Verification items for the finished model (mm, model axes). A direction names the side the tool comes from. Give positions to 0.01 mm unless a question says otherwise; leave off trailing zeros. Write each loop counter-clockwise with the first axis right and the second up, starting at its lowest first coordinate (ties: lowest second). Pieces come first, ordered by that corner, then holes. Notation, with made-up numbers: (8.25, -11.75) -> (44.25, -11.75) arc R22 ccw to (44.25, -0.75) -> close; hole circle Ø11 at (16, 11.25). An arc over 180 degrees is marked (long way). Answer as CSV lines item,"result".
```python
from build123d import *

# Parameters (mm, degrees)
SKETCH2_R          = 1.27
CUT_EXTRUDE1_DEPTH = 27.94
SKETCH3_R          = 2.54
CUT_EXTRUDE5_DEPTH = 2.54
CIRPATTERN1_COUNT  = 5


with BuildPart() as part:
    # Sketch1 → Revolve1 (revolve)
    with BuildSketch(Plane.YZ, mode=Mode.PRIVATE) as revolve1_sk:
        Polygon((0, 33.880456026), (-45.72, 33.880456026), (-45.72, 14.830456026), (-38.1, 14.830456026), (-38.1, 2.130456026), (0, 2.130456026), align=None)
    revolve(revolve1_sk.sketch.rotate(Axis((0, 0, 48.959120521), (0, 0, -1)), 270), axis=Axis((0, 0, 48.959120521), (0, 0, -1)))

    # Sketch2 → Cut-Extrude1 (cut)
    with BuildSketch(Plane.XY.offset(33.880456026)):
        with Locations((0, 41.91)):
            Circle(SKETCH2_R)
    cut_extrude1 = extrude(amount=-CUT_EXTRUDE1_DEPTH, mode=Mode.SUBTRACT)

    # Sketch3 → Cut-Extrude5 (cut)
    with BuildSketch(Plane.XY.offset(33.880456026)):
        with Locations((0, 41.91)):
            Circle(SKETCH3_R)
    cut_extrude5 = extrude(amount=-CUT_EXTRUDE5_DEPTH, mode=Mode.SUBTRACT)

    # CirPattern1: Cut-Extrude1, Cut-Extrude5 ×5 about axis
    cirpattern1_axis = Axis((0, 0, 0), (0, 0, 1))
    add([cut_extrude1.rotate(cirpattern1_axis, i * 360 / CIRPATTERN1_COUNT) for i in range(1, CIRPATTERN1_COUNT)], mode=Mode.SUBTRACT)
    add([cut_extrude5.rotate(cirpattern1_axis, i * 360 / CIRPATTERN1_COUNT) for i in range(1, CIRPATTERN1_COUNT)], mode=Mode.SUBTRACT)


solid = part.part
```
1) Section check C-C (z = 22.5). Record the boundary of the cut face in (x, y).
Reported:
outline,"circle Ø91.44 at (0, 0); hole circle Ø2.54 at (-39.86, 12.95); hole circle Ø2.54 at (-24.63, -33.91); hole circle Ø2.54 at (0, 41.91); hole circle Ø2.54 at (24.63, -33.91); hole circle Ø2.54 at (39.86, 12.95)"
2) Section check B-B (y = 0). Record the boundary of the cut face in (x, z), and give its area (3 significant figures).
Reported:
outline,"(-45.72, 14.83) -> (-38.1, 14.83) -> (-38.1, 2.13) -> (38.1, 2.13) -> (38.1, 14.83) -> (45.72, 14.83) -> (45.72, 33.88) -> (-45.72, 33.88) -> close"
area,"2,710 mm²"
3) Section check A-A (x = 0). Record the boundary of the cut face in (y, z), and give its area (3 significant figures).
Reported:
outline,"(-45.72, 14.83) -> (-38.1, 14.83) -> (-38.1, 2.13) -> (38.1, 2.13) -> (38.1, 14.83) -> (40.64, 14.83) -> (40.64, 31.34) -> (39.37, 31.34) -> (39.37, 33.88) -> (-45.72, 33.88) -> close; (43.18, 14.83) -> (45.72, 14.83) -> (45.72, 33.88) -> (44.45, 33.88) -> (44.45, 31.34) -> (43.18, 31.34) -> close"
area,"2,650 mm²"
4) Section check D-D (y = 41.91). Record the boundary of the cut face in (x, z).
Reported:
outline,"(-18.27, 14.83) -> (-1.27, 14.83) -> (-1.27, 31.34) -> (-2.54, 31.34) -> (-2.54, 33.88) -> (-18.27, 33.88) -> close; (1.27, 14.83) -> (18.27, 14.83) -> (18.27, 33.88) -> (2.54, 33.88) -> (2.54, 31.34) -> (1.27, 31.34) -> close"
5) Depth check by flat-ended pin: pin 1 (1.5 mm diameter, centred on x = 39.86, y = 12.95, fed in from +Z); pin 2 (5 mm diameter, centred on x = -14, z = 23.5, fed in from +Y); pin 3 (10 mm diameter, centred on x = -34, z = 29.5, fed in from -Y); pin 4 (1.5 mm diameter, centred on x = -13, z = 6, fed in from -Y). Enter the tip coordinate at first touch or a pass-through.
Reported:
pin 1,"through"
pin 2,"y = 44.25"
pin 3,"y = -35.35"
pin 4,"y = -36.08"
6) Draft check along X on faces 4 (the cylindrical face through (-30.235, 23.183, 8.392)), 5 (the flat face through (-1, -1, 2.13)), 6 (the flat face through (-41, 14, 31.34)). Enter one of: +X half, -X half, draft (parallel to the pull), parting line (faces both ways), or undercut.
Reported:
face 4,"parting line"
face 5,"draft"
face 6,"undercut"
7) Tool access check on faces 1 (the cylindrical face through (-24.45, -32.65, 23.2)), 2 (the flat face through (-27.3, -27.3, 14.83)), 3 (the flat face through (1, 43, 31.34)). Record the directions out of +Z, -Z, +X, -X, +Y, -Y that give a thin tool (end or side, any length) a straight path to the whole face; none if there is none.
Reported:
face 1,"+Z, -Z"
face 2,"-Z"
face 3,"+Z"
8) Scan lines: line 1 along X through (y, z) = (-35, 30); line 2 along X through (y, z) = (-33, 26); line 3 along X through (y, z) = (41, 19). Record each from-to range of solid material in increasing order.
Reported:
line 1,"-29.42 to -25.28, -23.99 to 23.99, 25.28 to 29.42"
line 2,"-31.64 to -25.52, -23.74 to 23.74, 25.52 to 31.64"
line 3,"-20.23 to -0.89, 0.89 to 20.23"
